from build123d import *

# Parameters (mm, degrees)
BOSS_EXTRUDE1_DEPTH = 15
SKETCH2_W           = 15
SKETCH2_H           = 32.5
BOSS_EXTRUDE2_DEPTH = 30
SKETCH3_W           = 10
SKETCH3_H           = 32.5
BOSS_EXTRUDE3_DEPTH = 30
SKETCH4_R           = 2.4
CUT_EXTRUDE1_DEPTH  = 5
CUT_EXTRUDE2_DEPTH  = 5
FILLET1_R           = 7
FILLET2_R           = 8
BOSS_EXTRUDE4_DEPTH = 5
SKETCH7_R           = 1.5
CUT_EXTRUDE3_DEPTH  = 6
FILLET3_R           = 2
FILLET4_R           = 1.5


with BuildPart() as part:
    # Sketch1 → Boss-Extrude1 (new body)
    with BuildSketch(Plane.XY):
        Polygon((-7.003618791, -14.915819089), (6.175, -14.915819089), (6.175, 7.584180911), (-7.003618791, 7.584180911), (-7.003618791, 12.584180911), (9.659757463, 12.584180911), (9.659757463, -19.915819089), (-7.003618791, -19.915819089), align=None)
    extrude(amount=BOSS_EXTRUDE1_DEPTH)

    # Sketch2 → Boss-Extrude2 (add)
    with BuildSketch(Plane(origin=(9.659757463, 0, 0), x_dir=(0, 0, -1), z_dir=(1, 0, 0))):
        with Locations((-7.5, -3.665819089)):
            Rectangle(SKETCH2_W, SKETCH2_H)
    extrude(amount=BOSS_EXTRUDE2_DEPTH)

    # Sketch3 → Boss-Extrude3 (add)
    with BuildSketch(Plane(origin=(0, 0, 0), x_dir=(-1, 0, 0), z_dir=(0, 0, -1))):
        with Locations((-34.659757463, -3.665819089)):
            Rectangle(SKETCH3_W, SKETCH3_H)
    extrude(amount=BOSS_EXTRUDE3_DEPTH)

    # Sketch4 → Cut-Extrude1 (cut)
    with BuildSketch(Plane(origin=(39.659757463, 0, 0), x_dir=(0, 0, -1), z_dir=(1, 0, 0))):
        with Locations((15, -3.53982496)):
            Circle(SKETCH4_R)
    extrude(amount=-CUT_EXTRUDE1_DEPTH, mode=Mode.SUBTRACT)

    # Sketch5 → Cut-Extrude2 (cut)
    with BuildSketch(Plane.XY.offset(15)):
        Polygon((39.659757463, 12.584180911), (-7.003618791, 12.584180911), (-7.003618791, 7.584180911), (6.175, 7.584180911), (6.175, -14.915819089), (-7.003618791, -14.915819089), (-7.003618791, -19.915819089), (39.659757463, -19.915819089), align=None)
    extrude(amount=-CUT_EXTRUDE2_DEPTH, mode=Mode.SUBTRACT)

    # Fillet1
    fillet1_edges = [part.edges().sort_by_distance(p)[0] for p in [
        (34.659757463, -19.915819089, -30),
        (34.659757463, 12.584180911, -30),
    ]]
    fillet(fillet1_edges, radius=FILLET1_R)

    # Fillet2
    fillet2_edges = [part.edges().sort_by_distance(p)[0] for p in [
        (29.659757463, -3.665819089, 0),
        (39.659757463, -3.665819089, 10),
    ]]
    fillet(fillet2_edges, radius=FILLET2_R)

    # Sketch6 → Boss-Extrude4 (add)
    with BuildSketch(Plane.ZY.offset(7.003618791)):
        with BuildLine():
            Line((0, 7.584180911), (10, 7.584180911))
            Line((10, 7.584180911), (10, 18.584180911))
            ThreePointArc((10, 18.584180911), (9.414213562, 19.998394474), (8, 20.584180911))
            Line((8, 20.584180911), (2, 20.584180911))
            ThreePointArc((2, 20.584180911), (0.585786438, 19.998394474), (0, 18.584180911))
            Line((0, 18.584180911), (0, 7.584180911))
        make_face()
        with BuildLine():
            Line((10, -14.915819089), (10, -25.915819089))
            ThreePointArc((10, -25.915819089), (9.414213562, -27.330032651), (8, -27.915819089))
            Line((8, -27.915819089), (2, -27.915819089))
            ThreePointArc((2, -27.915819089), (0.585786438, -27.330032651), (0, -25.915819089))
            Line((0, -25.915819089), (0, -14.915819089))
            Line((0, -14.915819089), (10, -14.915819089))
        make_face()
    extrude(amount=-BOSS_EXTRUDE4_DEPTH)

    # Sketch7 → Cut-Extrude3 (cut, through all)
    with BuildSketch(Plane(origin=(-2.003618791, 0, 0), x_dir=(0, 0, -1), z_dir=(1, 0, 0))):
        with Locations((-5, -23.915819089)):
            Circle(SKETCH7_R)
        with Locations((-5, 16.584180911)):
            Circle(SKETCH7_R)
    extrude(amount=-CUT_EXTRUDE3_DEPTH, mode=Mode.SUBTRACT)

    # Fillet3
    fillet3_edges = [part.edges().sort_by_distance(p)[0] for p in [
        (14.828069336, 12.584180911, 10),
        (9.828069336, 12.584180911, 0),
        (37.316611713, 12.584180911, 7.656854249),
        (39.659757463, -19.915819089, -10.5),
        (37.316611713, -19.915819089, 7.656854249),
        (27.316611713, 12.584180911, -2.343145751),
        (27.316611713, -19.915819089, -2.343145751),
        (14.828069336, -19.915819089, 10),
        (9.828069336, -19.915819089, 0),
        (39.659757463, -3.665819089, -30),
        (29.659757463, -3.665819089, -30),
        (39.659757463, 12.584180911, -10.5),
        (39.659757463, -17.865566557, -27.949747468),
        (39.659757463, 10.53392838, -27.949747468),
        (29.659757463, 12.584180911, -15.5),
        (29.659757463, -19.915819089, -15.5),
        (29.659757463, -17.865566557, -27.949747468),
        (29.659757463, 10.53392838, -27.949747468),
    ]]
    fillet(fillet3_edges, radius=FILLET3_R)

    # Fillet4
    fillet4_edges = [part.edges().sort_by_distance(p)[0] for p in [
        (-2.003618791, 15.584180911, 0),
        (-2.003618791, 15.584180911, 10),
        (-2.003618791, 19.998394474, 0.585786438),
        (-2.003618791, 20.584180911, 5),
        (-2.003618791, 19.998394474, 9.414213562),
        (-2.003618791, -22.915819089, 10),
        (-2.003618791, -22.915819089, 0),
        (-2.003618791, -27.330032651, 9.414213562),
        (-2.003618791, -27.915819089, 5),
        (-2.003618791, -27.330032651, 0.585786438),
    ]]
    fillet(fillet4_edges, radius=FILLET4_R)


solid = part.part
Verification items for the finished model (mm, model axes). A direction names the side the tool comes from. Coordinates: 2 decimals unless noted, no trailing zeros. Order: outer loops, then holes, each group sorted by start corner. A loop starts at its lowest first (then second) coordinate and runs counter-clockwise, first axis right, second up.
Item 1: Release check for a two-part mould opening along Z. For faces 5 (the face through (39.66, -7, -13)), 6 (the face through (34.66, -4, -15)), 7 (the face through (-5.28, 19.98, 9.43)) record: +Z half, -Z half, draft (parallel to the pull), parting line (faces both ways), or undercut.
Filled in:
face 5: draft
face 6: undercut
face 7: +Z half
Item 2: Section check B-B, the plane y = 4. Enter the section's corners in (x, z) (3 decimals), then the cut area to 3 significant figures.
Filled in:
outline: (6.175, 0) - (21.66, 0) arc R8 cw to (29.66, -8) - (29.66, -28) arc R2 ccw to (31.66, -30) - (37.66, -30) arc R2 ccw to (39.66, -28) - (39.66, 2) arc R8 ccw to (31.66, 10) - (6.175, 10) - close
area: 633 mm2
Item 3: Section check D-D, the plane x = 19.5. Enter the section's corners in (y, z), then the cut area to 3 significant figures.
Filled in:
outline: (-19.92, 2) arc R2 ccw to (-17.92, 0) - (10.58, 0) arc R2 ccw to (12.58, 2) - (12.58, 8) arc R2 ccw to (10.58, 10) - (-17.92, 10) arc R2 ccw to (-19.92, 8) - close
area: 322 mm2
Item 4: Material ranges on L1, parallel to Y at x = 3.5, z = 4.5; L2, parallel to Y at x = 37.1, z = -15; L3, parallel to Z at x = 11.5, y = -5.5, recorded low to high.
Filled in:
L1: y = -19.92 to -14.92, 7.58 to 12.58
L2: y = -19.92 to -5.94, -1.14 to 12.58
L3: z = 0 to 10
Item 5: Section check C-C, the plane z = -15. Enter the section's corners in (x, y).
Filled in:
outline: (29.66, -17.92) arc R2 ccw to (31.66, -19.92) - (37.66, -19.92) arc R2 ccw to (39.66, -17.92) - (39.66, -5.94) - (34.66, -5.94) - (34.66, -1.14) - (39.66, -1.14) - (39.66, 10.58) arc R2 ccw to (37.66, 12.58) - (31.66, 12.58) arc R2 ccw to (29.66, 10.58) - close
Item 6: Depth check by flat-ended pin: pin 1 (10 mm diameter, centred on y = 0, z = -14.5, fed in from -X); pin 2 (1.5 mm diameter, centred on x = 21.5, z = -2.5, fed in from -Y); pin 3 (3 mm diameter, centred on y = -0.5, z = 4.5, fed in from -X) (3 decimals); pin 4 (10 mm diameter, centred on x = 27, z = 2.5, fed in from +Y). Enter the tip coordinate at first touch or a pass-through.
Filled in:
pin 1: stops at x = 29.66
pin 2: passes through
pin 3: stops at x = 6.175
pin 4: stops at y = 12.58
Item 7: Section check A-A, the plane x = 4. Enter the section's corners in (y, z).
Filled in:
outline: (-19.92, 2) arc R2 ccw to (-17.92, 0) - (-14.92, 0) - (-14.92, 10) - (-17.92, 10) arc R2 ccw to (-19.92, 8) - close; (7.58, 0) - (10.58, 0) arc R2 ccw to (12.58, 2) - (12.58, 8) arc R2 ccw to (10.58, 10) - (7.58, 10) - close
Item 8: Access from +Z, -Z, +X, -X, +Y, -Y to the whole of each face (thin tool, end or side, straight path). Record for faces 1 (the face through (8.9, 12.01, 0.6)), 2 (the face through (-1, -14.916, 5)), 3 (the face through (25, 12.584, 3)), 4 (the face through (37.195, -3.434, -12.602)).
Filled in:
face 1: -Z, +Y
face 2: +Z, -Z, -X
face 3: +Z, -Z, +X, +Y
face 4: +X
